Part print with two shaded views. Sizes in mm from the minimum x, y, z corner. A direction names the side the tool comes from. Round coordinates to 2 decimals unless told otherwise and drop trailing zeros. Write each loop counter-clockwise with the first axis right and the second up, starting at its lowest first coordinate (ties: lowest second). Pieces come first, ordered by that corner, then holes. Notation, with made-up numbers: M 64,-30.75 L 88,-30.75 A18 ccw 88,-4.75 Z; hole C 87,40.5 d7. An arc over 180 degrees is marked long. Use one line per item in the form item = value. Start each with the question number.
Item 1: Cut at C-C, the plane z = 15. Give the cut face in (x, y).
Item 2: Cut at D-D, the plane x = 0.9. Give the cut face in (y, z).
Item 3: Mould opens along Y. For the marked faces 3, 4 and 5 say: +Y half, -Y half, draft (parallel to the pull), parting line (faces both ways), or undercut.
Item 4: Flat gauge pin, fed straight in: pin 1 Ø3 at (x, z) = (1, 5.5) entering from -Y. Where does the tip first touch, or does it go through?
Item 5: Cut at A-A, the plane z = 2.25. Give the cut face in (x, y), then the cut area to 3 significant figures.
Item 6: Cut at B-B, the plane y = 0.7. Give the cut face in (x, z).
Item 7: Which spindle directions (+Z, -Z, +X, -X, +Y, -Y) get a long thin tool onto all of the face, cutting with end or side? Do the marked faces 1 and 2. Say none if no direction does.
Item 8: Probe L1, parallel to Y at x = 3, z = 21.5; L2, parallel to X at y = 3.35, z = 24; L3, parallel to Y at x = 2.4, z = 22.5 (1 decimal). List the from-to ranges inside material, lowest first.
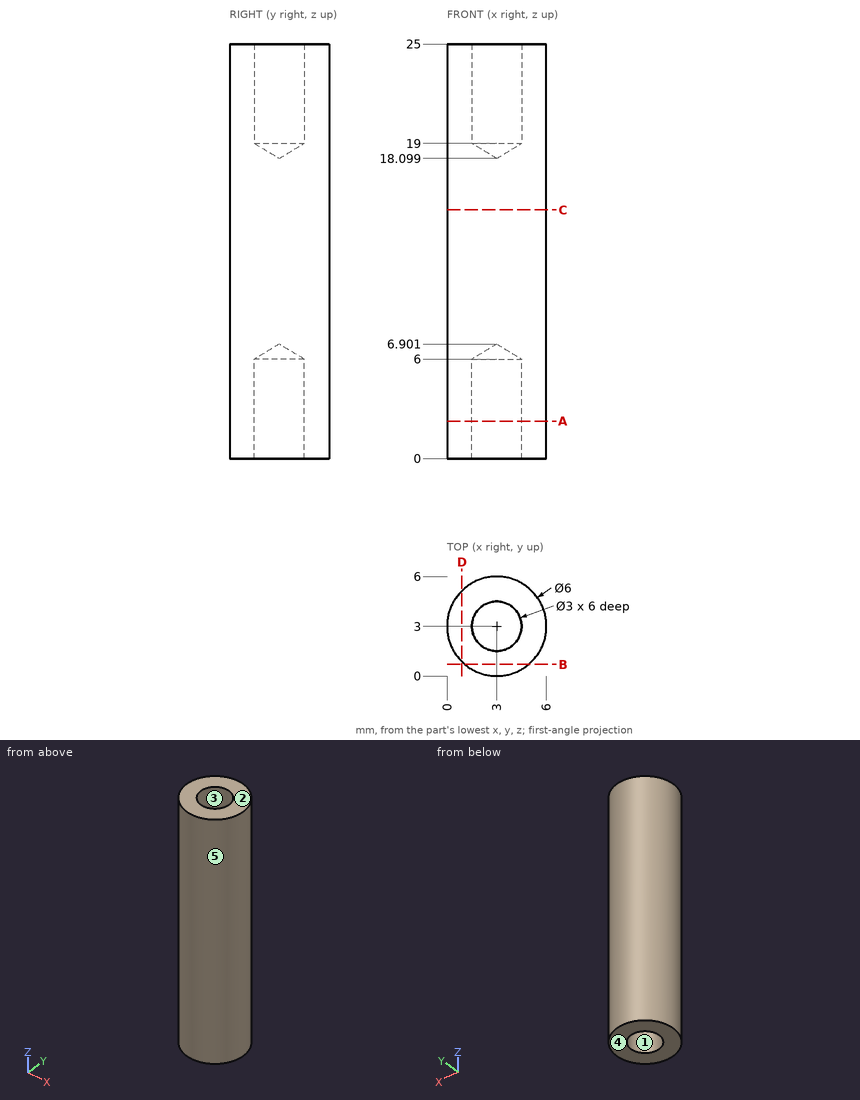
Model answer:
q1.outline = C 3,3 d6
q2.outline = M 0.86,0 L 5.14,0 L 5.14,25 L 0.86,25 Z
q3.face_3 = undercut
q3.face_4 = draft
q3.face_5 = parting line
q4.pin_1 = 0.04
q5.outline = C 3,3 d6; hole C 3,3 d3
q5.area = 21.2 mm²
q6.outline = M 1.07,0 L 4.93,0 L 4.93,25 L 1.07,25 Z
q7.face_1 = -Z
q7.face_2 = +Z, +X, -X, +Y, -Y
q8.L1 = 0 to 1.5, 4.5 to 6
q8.L2 = 0.02 to 1.54, 4.46 to 5.98
q8.L3 = 0.1 to 1.6, 4.4 to 5.9
